Autodesk Inventor part; units mm, degrees
ref_plane "YZ Plane" through (0, 0, 0) normal (1, 0, 0) x (0, 1, 0)
ref_plane "XZ Plane" through (0, 0, 0) normal (0, 1, 0) x (-1, 0, 0)
ref_plane "XY Plane" through (0, 0, 0) normal (0, 0, 1) x (1, 0, 0)
sketch "Sketch1" plane through (0, 0, 0) normal (0, 0, 1) x (1, 0, 0)
  line L0 (0, 0) -> (29, 0)
  line L1 (29, 0) -> (29, 21)
  line L2 (29, 21) -> (0, 21)
  line L3 (0, 21) -> (0, 0)
  dimension "d0" = 29
  dimension "d1" = 21
extrude "Extrusion1" add sketch "Sketch1" along normal blind 20
sketch "Sketch2" plane through (29, 0, 0) normal (1, 0, 0) x (0, 0, -1)
  line L0 (-7, 4) -> (-14, 4)
  line L1 (-14, 4) -> (-14, 17)
  line L2 (-14, 17) -> (-7, 17)
  line L3 (-7, 17) -> (-7, 4)
  line L4 (-20, 0) -> (-20, 21) construction
  line L5 (-14, 7) -> (-15.5, 7)
  line L6 (-15.5, 7) -> (-15.5, 14)
  line L7 (-15.5, 14) -> (-14, 14)
  line L8 (-14, 14) -> (-14, 7)
  line L9 (-15.5, 17) -> (-7, 17)
  line L10 (0, 21) -> (-20, 21) construction
  line L11 (-15.5, 12.5) -> (-16.5, 12.5)
  line L12 (-16.5, 12.5) -> (-16.5, 8.5)
  line L13 (-16.5, 8.5) -> (-15.5, 8.5)
  line L14 (-15.5, 8.5) -> (-15.5, 12.5)
  line L15 (0, 0) -> (0, 21)
  point P0 (-14, 10.5)
  point P1 (-20, 10.5)
  point P2 (-11.25, 17)
  point P3 (-10, 21)
  point P4 (-15.5, 10.5)
  dimension "d4" = 7
  dimension "d5" = 13
  dimension "d6" = 1.5
  dimension "d7" = 7
  dimension "d12" = 4
  dimension "d13" = 1
  dimension "d14" = 7
extrude "Extrusion2" cut sketch "Sketch2" against normal blind 12.7
sketch "Sketch3" plane through (0, 0, 0) normal (-1, 0, 0) x (0, 0, 1)
  line L0 (14, 14) -> (14, 17)
  line L1 (15.5, 14) -> (14, 14)
  line L2 (15.5, 7) -> (15.5, 14)
  line L3 (14, 7) -> (15.5, 7)
  line L4 (7, 4) -> (14, 4)
  line L5 (7, 17) -> (7, 4)
  line L6 (14, 17) -> (7, 17)
  line L7 (14, 4) -> (14, 7)
  point P0 (0, 0)
extrude "Extrusion3" cut sketch "Sketch3" against normal blind 12.7
sketch "Sketch4" plane through (29, 0, 0) normal (1, 0, 0) x (0, 0, -1)
  line L0 (-18, 3) -> (-3, 3)
  line L1 (-3, 3) -> (-3, 18)
  line L2 (-3, 18) -> (-18, 18)
  line L3 (-18, 18) -> (-18, 3)
  line L4 (-20, 0) -> (-20, 21)
  line L5 (-15.5, 8.5) -> (-16.5, 8.5)
  line L6 (-15.5, 7) -> (-15.5, 8.5)
  line L7 (-14, 7) -> (-15.5, 7)
  line L8 (-14, 4) -> (-14, 7)
  line L9 (-7, 4) -> (-14, 4)
  line L10 (-7, 17) -> (-7, 4)
  line L11 (-14, 17) -> (-7, 17)
  line L12 (-14, 14) -> (-14, 17)
  line L13 (-15.5, 14) -> (-14, 14)
  line L14 (-15.5, 12.5) -> (-15.5, 14)
  line L15 (-16.5, 12.5) -> (-15.5, 12.5)
  line L16 (-16.5, 8.5) -> (-16.5, 12.5)
  point P0 (0, 0)
  point P1 (-18, 10.5)
  point P2 (-20, 10.5)
  dimension "d15" = 15
  dimension "d16" = 15
  dimension "d17" = 2
extrude "Extrusion4" add sketch "Sketch4" along normal blind 0.1
fillet "Fillet1" radius 2 4 edges at (14.5, 0, 0) (14.5, 0, 20) (14.5, 21, 20) (14.5, 21, 0)
properties part number "Ethernet Port" material "ABS Plastic"
The listing builds one solid part. Answer for the finished solid, in the listing's coordinates (mm). A direction names the side the tool comes from. Give positions to 0.01 mm unless a question says otherwise; leave off trailing zeros. Order: outer loops, then holes, each group sorted by start corner. A loop starts at its lowest first (then second) coordinate and runs counter-clockwise, first axis right, second up. Notation, with made-up numbers: (45, -33) - (81, -33) arc R7 cw to (81, -25) - close; hole circle Ø4 at (-32, -20.5). An arc over 180 degrees is marked (long way). Use one line per item in the form item = value.
1) Consider probe 1 along Z at (x, y) = (9.75, 10.5); probe 2 along Y at (x, z) = (23.75, 11); probe 3 along Y at (x, z) = (2.5, 14.25). Determine where each line is inside the solid, lowest interval first. Write a range as [from, to].
Verdict:
probe_1 = [0, 7], [15.5, 20]
probe_2 = [0, 4], [17, 21]
probe_3 = [0, 7], [14, 21]
2) Find section D-D on x = 23.75. Determine the outline of the cut face in (y, z).
Verdict:
outline = (0, 2) arc R2 ccw to (2, 0) - (19, 0) arc R2 ccw to (21, 2) - (21, 18) arc R2 ccw to (19, 20) - (2, 20) arc R2 ccw to (0, 18) - close; hole (4, 7) - (17, 7) - (17, 14) - (14, 14) - (14, 15.5) - (12.5, 15.5) - (12.5, 16.5) - (8.5, 16.5) - (8.5, 15.5) - (7, 15.5) - (7, 14) - (4, 14) - close
3) The mould has two halves that part along Z. Classify faces 4 (the flat face through (6, 10, 15.5)), 5 (the cylindrical face through (14.3, 20.43, 0.6)), 6 (the flat face through (29.1, 11, 6)): released by +Z, released by -Z, zero draft, split by the parting line, or undercut.
Verdict:
face_4 = undercut
face_5 = released by -Z
face_6 = zero draft
4) Find section A-A on x = 5.5. Determine the outline of the cut face in (y, z), and give its area (3 significant figures).
Verdict:
outline = (0, 2) arc R2 ccw to (2, 0) - (19, 0) arc R2 ccw to (21, 2) - (21, 18) arc R2 ccw to (19, 20) - (2, 20) arc R2 ccw to (0, 18) - close; hole (4, 7) - (17, 7) - (17, 14) - (14, 14) - (14, 15.5) - (7, 15.5) - (7, 14) - (4, 14) - close
area = 315 mm^2
5) For faces 1 (the flat face through (23, 8, 15.5)), 2 (the cylindrical face through (14.7, 0.6, 19.43)), 3 (the flat face through (6, 4, 10)), determine the directions among +Z, -Z, +X, -X, +Y, -Y from which every point of the face is accessible in a straight line to the end or side of a thin tool.
Verdict:
face_1 = +X
face_2 = +Z, +X, -X, -Y
face_3 = -X
6) Find section B-B on z = 10. Determine the outline of the cut face in (x, y).
Verdict:
outline = (0, 0) - (29, 0) - (29, 3) - (29.1, 3) - (29.1, 4) - (16.3, 4) - (16.3, 17) - (29.1, 17) - (29.1, 18) - (29, 18) - (29, 21) - (0, 21) - (0, 17) - (12.7, 17) - (12.7, 4) - (0, 4) - close
7) Find section C-C on y = 11. Determine the outline of the cut face in (x, z).
Verdict:
outline = (0, 0) - (29, 0) - (29, 3) - (29.1, 3) - (29.1, 7) - (16.3, 7) - (16.3, 16.5) - (29.1, 16.5) - (29.1, 18) - (29, 18) - (29, 20) - (0, 20) - (0, 15.5) - (12.7, 15.5) - (12.7, 7) - (0, 7) - close
